Autodesk Inventor part; units mm, degrees
ref_plane "YZ Plane" through (0, 0, 0) normal (1, 0, 0) x (0, 1, 0)
ref_plane "XZ Plane" through (0, 0, 0) normal (0, 1, 0) x (-1, 0, 0)
ref_plane "XY Plane" through (0, 0, 0) normal (0, 0, 1) x (1, 0, 0)
sketch "Sketch1" plane through (0, 0, 0) normal (0, 0, 1) x (1, 0, 0)
  circle A0 centre (-18.2965, -47.165) radius 1.2295 construction
  circle A1 centre (-6.0724, -26.0926) radius 1.2295 construction
  circle A2 centre (5.6859, -42.8853) radius 1.2295 construction
  circle A3 centre (-0.1932, -34.489) radius 6 construction
  circle A4 centre (-7.5, -9) radius 1.621 construction
  circle A5 centre (-10.5, 0) radius 2.067 construction
  circle A6 centre (-7.5, 9) radius 1.621 construction
  circle A7 centre (-35, 0) radius 4 construction
  circle A8 centre (-62.5, 9) radius 1.621 construction
  line L0 (-55, -16) -> (-55, 16) construction
  circle A9 centre (-65.5, 0) radius 2.067 construction
  circle A10 centre (-62.5, -9) radius 1.621 construction
  circle A11 centre (-65.5, 0) radius 2.067 construction
  circle A12 centre (-62.5, 9) radius 1.7295 construction
  circle A13 centre (-62.5, -9) radius 1.7295 construction
  line L1 (-70, 13.1624) -> (-55, 13.1624) construction
  line L2 (-70, -13.1624) -> (-70, 13.1624) construction
  line L3 (-55, -13.1624) -> (-70, -13.1624) construction
  line L4 (-55, 13.1624) -> (-55, -13.1624) construction
  circle A14 centre (-10.5, 0) radius 2.067 construction
  circle A15 centre (-7.5, -9) radius 1.621 construction
  circle A16 centre (-7.5, 9) radius 1.621 construction
  line L5 (-15, 13.1624) -> (0, 13.1624) construction
  line L6 (-15, -13.1624) -> (-15, 13.1624) construction
  line L7 (0, -13.1624) -> (-15, -13.1624) construction
  line L8 (0, 13.1624) -> (0, -13.1624) construction
  arc A17 (4.363, -44.1343) -> (4.0127, -42.1709) centre (-18.2965, -47.165) ccw
  arc A18 (7.3366, -43.7366) -> (6.9402, -41.5156) centre (-18.2965, -47.165) ccw
  arc A19 (-5.9734, -27.9093) -> (-7.6985, -26.9086) centre (-18.2965, -47.165) ccw
  arc A20 (-4.3563, -25.3825) -> (-6.3078, -24.2504) centre (-18.2965, -47.165) ccw
  arc A21 (-4.9287, -38.6488) -> (-5.7218, -37.5161) centre (-18.2965, -47.165) ccw
  arc A22 (5.6137, -31.9325) -> (4.1951, -29.9066) centre (-18.2965, -47.165) ccw
  arc A23 (-5.1648, -26.6459) -> (-7.0032, -25.5795) centre (-18.2965, -47.165) ccw construction
  arc A24 (0.3425, -35.2907) -> (-0.7634, -33.7114) centre (-18.2965, -47.165) ccw construction
  arc A25 (5.8498, -43.9354) -> (5.4764, -41.8432) centre (-18.2965, -47.165) ccw construction
  arc A26 (6.9402, -41.5156) -> (4.0127, -42.1709) centre (5.4764, -41.8432) ccw
  arc A27 (4.363, -44.1343) -> (7.3366, -43.7366) centre (5.8498, -43.9354) ccw
  arc A28 (-4.9287, -38.6488) -> (5.6137, -31.9325) centre (0.3425, -35.2907) ccw
  arc A29 (4.1951, -29.9066) -> (-5.7218, -37.5161) centre (-0.7634, -33.7114) ccw
  arc A30 (-5.9734, -27.9093) -> (-4.3563, -25.3825) centre (-5.1648, -26.6459) ccw
  arc A31 (-6.3078, -24.2504) -> (-7.6985, -26.9086) centre (-7.0032, -25.5795) ccw
  circle A32 centre (-18.2965, -47.165) radius 1.5
  circle A33 centre (-7.5, -9) radius 2
  circle A34 centre (-7.5, 9) radius 2
  circle A35 centre (-10.5, 0) radius 2.5
  circle A36 centre (-62.5, 9) radius 2
  circle A37 centre (-65.5, 0) radius 2.5
  circle A38 centre (-62.5, -9) radius 2
  circle A39 centre (-7.3444, -39.4963) radius 17.7 construction
  arc A40 (-16.3879, -54.7116) -> (6.7463, -28.7846) centre (-7.3444, -39.4963) ccw
  arc A41 (0, -8.7624) -> (6.7463, -28.7846) centre (33.0845, -8.7624) ccw
  line L9 (0, -8.7624) -> (0, 9.1624)
  line L10 (-11, 13.1624) -> (-4, 13.1624)
  line L11 (-15, 9.1624) -> (-15, 0)
  line L12 (-55, 0) -> (-55, 9.1624)
  line L13 (-66, 13.1624) -> (-59, 13.1624)
  line L14 (-70, 9.1624) -> (-70, -13.1624)
  arc A42 (-55, 0) -> (-15, 0) centre (-35, 0) ccw
  arc A43 (-66, 13.1624) -> (-70, 9.1624) centre (-66, 9.1624) ccw
  arc A44 (-55, 9.1624) -> (-59, 13.1624) centre (-59, 9.1624) ccw
  arc A45 (-11, 13.1624) -> (-15, 9.1624) centre (-11, 9.1624) ccw
  arc A46 (0, 9.1624) -> (-4, 13.1624) centre (-4, 9.1624) ccw
  line L15 (-61.6755, -27.7942) -> (-16.3879, -54.7116)
  arc A47 (-70, -13.1624) -> (-61.6755, -27.7942) centre (-52.9789, -13.1624) ccw
  arc A48 (-35.0864, -30.8138) -> (-21.0883, -27.4948) centre (-35, 0) ccw
  line L16 (-35.0864, -30.8138) -> (-21.3261, -38.9925)
  line L17 (-15.2824, -31.0639) -> (-15.2824, -35.554)
  arc A49 (-15.2824, -31.0639) -> (-21.0883, -27.4948) centre (-19.2824, -31.0639) ccw
  arc A50 (-21.3261, -38.9925) -> (-15.2824, -35.554) centre (-19.2824, -35.554) ccw
  point P0 (0, 0)
  point P1 (-15.2824, -23.6794)
  dimension "d0" = 3
  dimension "d1" = 5
  dimension "d2" = 5
  dimension "d3" = 5
  dimension "d4" = 12.5
  dimension "d5" = 3
  dimension "d6" = 4
  dimension "d7" = 4
  dimension "d8" = 5
  dimension "d9" = 4
  dimension "d10" = 5
  dimension "d11" = 4
  dimension "d12" = 4
  dimension "d15" = 4
extrude "Extrusion1" add sketch "Sketch1" along normal blind 3
sketch "Sketch2" plane through (0, 0, 3) normal (0, 0, 1) x (1, 0, 0)
  arc A0 (4.1951, -29.9066) -> (-5.7218, -37.5161) centre (-0.7634, -33.7114) ccw
  arc A1 (5.6137, -31.9325) -> (4.1951, -29.9066) centre (-18.2965, -47.165) ccw
  arc A2 (-4.9287, -38.6488) -> (5.6137, -31.9325) centre (0.3425, -35.2907) ccw
  arc A3 (-4.9287, -38.6488) -> (-5.7218, -37.5161) centre (-18.2965, -47.165) ccw
  arc A4 (-35.0864, -30.8138) -> (-21.0883, -27.4948) centre (-35, 0) ccw
  arc A5 (-15.2824, -31.0639) -> (-21.0883, -27.4948) centre (-19.2824, -31.0639) ccw
  line L0 (-15.2824, -31.0639) -> (-15.2824, -35.554)
  arc A6 (-21.3261, -38.9925) -> (-15.2824, -35.554) centre (-19.2824, -35.554) ccw
  line L1 (-21.3261, -38.9925) -> (-35.0864, -30.8138)
  circle A7 centre (-65.5, 0) radius 2.5
  circle A8 centre (-10.5, 0) radius 2.5
  arc A9 (-6.3078, -24.2504) -> (-7.6985, -26.9086) centre (-7.0032, -25.5795) ccw
  arc A10 (-4.3563, -25.3825) -> (-6.3078, -24.2504) centre (-18.2965, -47.165) ccw
  arc A11 (-5.9734, -27.9093) -> (-4.3563, -25.3825) centre (-5.1648, -26.6459) ccw
  arc A12 (-5.9734, -27.9093) -> (-7.6985, -26.9086) centre (-18.2965, -47.165) ccw
  arc A13 (6.9402, -41.5156) -> (4.0127, -42.1709) centre (5.4764, -41.8432) ccw
  arc A14 (7.3366, -43.7366) -> (6.9402, -41.5156) centre (-18.2965, -47.165) ccw
  arc A15 (4.363, -44.1343) -> (7.3366, -43.7366) centre (5.8498, -43.9354) ccw
  arc A16 (4.363, -44.1343) -> (4.0127, -42.1709) centre (-18.2965, -47.165) ccw
  circle A17 centre (-62.5, -9) radius 2
  circle A18 centre (-62.5, 9) radius 2
  circle A19 centre (-7.5, 9) radius 2
  circle A20 centre (-7.5, -9) radius 2
  circle A21 centre (-18.2965, -47.165) radius 1.5
  line L2 (-70, 9.1624) -> (-70, -13.1624)
  arc A22 (-70, -13.1624) -> (-61.6755, -27.7942) centre (-52.9789, -13.1624) ccw
  line L3 (-61.6755, -27.7942) -> (-16.3879, -54.7116)
  arc A23 (-16.3879, -54.7116) -> (6.7463, -28.7846) centre (-7.3444, -39.4963) ccw
  arc A24 (0, -8.7624) -> (6.7463, -28.7846) centre (33.0845, -8.7624) ccw
  line L4 (0, -8.7624) -> (0, 9.1624)
  arc A25 (0, 9.1624) -> (-4, 13.1624) centre (-4, 9.1624) ccw
  line L5 (-4, 13.1624) -> (-11, 13.1624)
  arc A26 (-11, 13.1624) -> (-15, 9.1624) centre (-11, 9.1624) ccw
  line L6 (-15, 9.1624) -> (-15, 0)
  arc A27 (-55, 0) -> (-15, 0) centre (-35, 0) ccw
  line L7 (-55, 0) -> (-55, 9.1624)
  arc A28 (-55, 9.1624) -> (-59, 13.1624) centre (-59, 9.1624) ccw
  line L8 (-59, 13.1624) -> (-66, 13.1624)
  arc A29 (-66, 13.1624) -> (-70, 9.1624) centre (-66, 9.1624) ccw
  circle A30 centre (-62.5, 9) radius 1
  circle A31 centre (-65.5, 0) radius 1.75
  circle A32 centre (-62.5, -9) radius 2
  circle A33 centre (-62.5, -9) radius 1.1893
  circle A34 centre (-62.5, 9) radius 2
  circle A35 centre (-65.5, 0) radius 2.5
  circle A36 centre (-18.2965, -47.165) radius 1
  circle A37 centre (-7.5, -9) radius 1
  circle A38 centre (-7.5, 9) radius 1
  circle A39 centre (-10.5, 0) radius 1.75
  arc A40 (3.4017, -30.5154) -> (-4.9285, -36.9074) centre (-0.7634, -33.7114) ccw
  arc A41 (4.7703, -32.4698) -> (3.4017, -30.5154) centre (-18.2965, -47.165) ccw
  arc A42 (-4.0853, -38.1115) -> (4.7703, -32.4698) centre (0.3425, -35.2907) ccw
  arc A43 (-4.0853, -38.1115) -> (-4.9285, -36.9074) centre (-18.2965, -47.165) ccw
  arc A44 (6.4523, -41.6248) -> (4.5006, -42.0617) centre (5.4764, -41.8432) ccw
  arc A45 (6.841, -43.8029) -> (6.4523, -41.6248) centre (-18.2965, -47.165) ccw
  arc A46 (4.8586, -44.068) -> (6.841, -43.8029) centre (5.8498, -43.9354) ccw
  arc A47 (4.8586, -44.068) -> (4.5006, -42.0617) centre (-18.2965, -47.165) ccw
  arc A48 (-4.6258, -25.8036) -> (-6.5396, -24.6934) centre (-18.2965, -47.165) ccw
  arc A49 (-6.5396, -24.6934) -> (-7.4667, -26.4655) centre (-7.0032, -25.5795) ccw
  arc A50 (-5.7039, -27.4882) -> (-7.4667, -26.4655) centre (-18.2965, -47.165) ccw
  arc A51 (-5.7039, -27.4882) -> (-4.6258, -25.8036) centre (-5.1648, -26.6459) ccw
  point P0 (0, 0)
  dimension "d16" = 3.5
  dimension "d17" = 2
  dimension "d20" = 2
  dimension "d21" = 2
  dimension "d22" = 2
  dimension "d23" = 3.5
  dimension "d25" = 1
  dimension "d26" = 0.5
  dimension "d27" = 0.5
extrude "Extrusion2" add sketch "Sketch2" against normal up to surface (3 mm away) contours A1 A2 A3 A0 | A7 | A8 | A10 A11 A12 A9 | A14 A15 A16 A13 | A17 | A18 | A19 | A20 | A21
fillet "Fillet1" radius 1 1 edges at (-35.0864, -30.8138, 1.5)
Geometry check sheet. Reference: the model listing, model coordinates, mm. A direction names the side the tool comes from. Round coordinates to 2 decimals unless told otherwise and drop trailing zeros. Order: outer loops, then holes, each group sorted by start corner. A loop starts at its lowest first (then second) coordinate and runs counter-clockwise, first axis right, second up. Notation, with made-up numbers: M 72.25,-31.5 L 110.25,-31.5 A20 cw 110.25,-7.5 Z; hole C -32,8 d7. An arc over 180 degrees is marked long. Answer in a Markdown table with one row per item.
(1) Tool access check on faces 1 (the face through (-17.25, -39, 1.48)), 2 (the face through (-13.86, 11.96, 1.48)). Record the directions out of +Z, -Z, +X, -X, +Y, -Y that give a thin tool (end or side, any length) a straight path to the whole face; none if there is none.
Responses:
| item | result |
|---|---|
| face 1 | +Z, -Z |
| face 2 | +Z, -Z, +Y |
(2) Go/stop test with flat-tipped pins: P1, Ø1.6, axis at x = -7.5, y = -9, coming from the +Z side; P2, Ø0.9, axis at y = 4, z = 2, coming from the +X side; P3, Ø1, axis at y = -14.5, z = 1, coming from the +X side; P4, Ø1.5, axis at y = -25.5, z = 2, coming from the +X side. Record where each tip stops, or that it passes through.
Responses:
| item | result |
|---|---|
| P1 | passes through |
| P2 | stops at x = 0 |
| P3 | stops at x = 0.59 |
| P4 | stops at x = 5 |
(3) Sectioned sample at B-B, the plane x = 2. Record the cut outline in (y, z), and give its area (3 significant figures).
Responses:
| item | result |
|---|---|
| outline | M -54.53,0 L -40.27,0 L -40.27,3 L -54.53,3 Z; M -29.25,0 L -20.09,0 L -20.09,3 L -29.25,3 Z |
| area | 70.2 mm² |
(4) Draft check along Y on faces 3 (the face through (-1.2, 12.02, 1.48)), 4 (the face through (5.279, -40.863, 1.521)). Enter one of: released by +Y, released by -Y, zero draft, split by the parting line, or undercut.
Responses:
| item | result |
|---|---|
| face 3 | released by +Y |
| face 4 | undercut |
(5) Sectioned sample at A-A, the plane y = -17.5. Record the cut outline in (x, z), and give its area (3 significant figures).
Responses:
| item | result |
|---|---|
| outline | M -69.44,0 L -44.68,0 L -44.68,3 L -69.44,3 Z; M -25.32,0 L 1.17,0 L 1.17,3 L -25.32,3 Z |
| area | 154 mm² |
(6) Scan lines: probe 1 along Y at (x, z) = (-7.5, 1.5); probe 2 along Y at (x, z) = (-62.5, 2.05); probe 3 along X at (y, z) = (-35, 1.55). Record each from-to range of solid material in increasing order. Write a range as from..to.
Responses:
| item | result |
|---|---|
| probe 1 | y = -57.2..-26.45, -24.71..-10, -8..8, 10..13.16 |
| probe 2 | y = -27.27..-10.19, -7.81..8, 10..13.16 |
| probe 3 | x = -49.55..-28.04, -15.28..-5.85, 5.58..9.77 |
(7) Sectioned sample at C-C, the plane z = 2.1. State how many separate pieces and enclosed holes the cut face has, and give its area (3 significant figures).
Responses:
| item | result |
|---|---|
| separate pieces | 1 |
| enclosed holes | 11 |
| area | 2,710 mm² |
(8) Sectioned sample at D-D, the plane x = -56. Record the cut outline in (y, z).
Responses:
| item | result |
|---|---|
| outline | M -31.17,0 L 11.81,0 L 11.81,3 L -31.17,3 Z |
